Work out the finished part from the listing and answer in its coordinate system (mm). A direction names the side the tool comes from. Coordinates: 2 decimals unless noted, no trailing zeros. Write each loop counter-clockwise with the first axis right and the second up, starting at its lowest first coordinate (ties: lowest second). Pieces come first, ordered by that corner, then holes. Notation, with made-up numbers: (35.5, -19) - (90.5, -19) arc R31 cw to (90.5, 8) - close; hole circle Ø9 at (85, -13.5). An arc over 180 degrees is marked (long way). Use a Markdown table: item, result. Add a question column.
(1) Find the intervals of material crossed by line 1 (Y direction, x = 0, z = 43) (3 decimals); line 2 (Y direction, x = -10, z = 2.8); line 3 (X direction, y = 3, z = 31.5), in increasing order. Write a range as from..to.
(2) The part is cut by section A-A, the plane y = 0. Give the vertices of the cut face in (x, z) (3 decimals), then the cut area to 3 significant figures.
(3) The part is cut by section C-C, the plane z = 30. Give the vertices of the cut face in (x, y) (3 decimals), then the cut area to 3 significant figures.
(4) The part is cut by section D-D, the plane z = 45.5. Give the vertices of the cut face in (x, y) (3 decimals).
(5) A tool of negligible diameter and unlimited length cuts with its end or side. For faces 4 (the face through (3, 0, 50)), 5 (the face through (0, 0, 40)), 6 (the face through (10, 0, 5)), from which of +Z, -Z, +X, -X, +Y, -Y can it reach the whole face along a straight path? Write none if from no direction.
(6) For a pull along Y with two mould halves and no side action, classify faces 1 (the face through (0, 0, 0)), 2 (the face through (8.75, -0.05, 2.46)), 3 (the face through (-3.441, -15.497, 24.65)) as released by +Y, released by -Y, zero draft, split by the parting line, or undercut.
(7) The part is cut by section B-B, the plane x = -10. Give the vertices of the cut face in (y, z), then the cut area to 3 significant figures.
(8) Given pin 1 Ø10 at (y, z) = (-1, 8.5) entering from +X (3 decimals); pin 2 Ø0.8 at (x, y) = (-10.5, -0.5) entering from -Z; pin 3 Ø1 at (x, z) = (1, 36) entering from +Y; pin 4 Ø5 at (x, z) = (-8, 38.5) entering from -Y, each flat-ended and moving along its own axis, determine where each tip first touches the part or whether it passes through.
from build123d import *

# Parameters (mm, degrees)
F0_R     = 15.875
F1_DEPTH = 50
F2_R     = 2.5
F3_DEPTH = 10
F4_R     = 1.25
F5_DEPTH = 5


with BuildPart() as f1:
    # F0 (on Top) → F1 (new body)
    with BuildSketch(Plane.XY):
        Circle(F0_R)
    extrude(amount=F1_DEPTH)

    # F2 (on face) → F3 (cut)
    with BuildSketch(Plane.XY.offset(50)):
        Circle(F2_R)
    extrude(amount=-F3_DEPTH, mode=Mode.SUBTRACT)

    # F4 (on face) → F5 (cut)
    with BuildSketch(Plane(origin=(0, 0, 0), x_dir=(1, 0, 0), z_dir=(0, 0, -1))):
        with Locations((10, 0)):
            Circle(F4_R)
        with Locations((-10, 0)):
            Circle(F4_R)
    extrude(amount=-F5_DEPTH, mode=Mode.SUBTRACT)


solid = f1.part
Model answer:
| question | item | result |
|---|---|---|
| 1 | line 1 | -15.875..-2.5, 2.5..15.875 |
| 1 | line 2 | -12.33..-1.25, 1.25..12.33 |
| 1 | line 3 | -15.59..15.59 |
| 2 | outline | (-15.875, 0) - (-11.25, 0) - (-11.25, 5) - (-8.75, 5) - (-8.75, 0) - (8.75, 0) - (8.75, 5) - (11.25, 5) - (11.25, 0) - (15.875, 0) - (15.875, 50) - (2.5, 50) - (2.5, 40) - (-2.5, 40) - (-2.5, 50) - (-15.875, 50) - close |
| 2 | area | 1,510 mm^2 |
| 3 | outline | circle Ø31.75 at (0, 0) |
| 3 | area | 792 mm^2 |
| 4 | outline | circle Ø31.75 at (0, 0); hole circle Ø5 at (0, 0) |
| 5 | face 4 | +Z, +X, -X, +Y, -Y |
| 5 | face 5 | +Z |
| 5 | face 6 | -Z |
| 6 | face 1 | zero draft |
| 6 | face 2 | undercut |
| 6 | face 3 | split by the parting line |
| 7 | outline | (-12.33, 0) - (-1.25, 0) - (-1.25, 5) - (1.25, 5) - (1.25, 0) - (12.33, 0) - (12.33, 50) - (-12.33, 50) - close |
| 7 | area | 1,220 mm^2 |
| 8 | pin 1 | x = 15.875 |
| 8 | pin 2 | z = 5 |
| 8 | pin 3 | y = 15.87 |
| 8 | pin 4 | y = -14.89 |
